Check sheet for the modelled part. Datum: model origin and axes. Units: mm. A direction names the side the tool comes from. Round coordinates to 2 decimals unless told otherwise and drop trailing zeros. Loops run counter-clockwise (first coordinate to the right, second up) from the corner with the lowest first, then second, coordinate; pieces in that order, holes last. Notation, with made-up numbers: (16, 31.5) -> (64, 31.5) arc R21 ccw to (64, 50.5) -> close; hole circle Ø7 at (24, -31). An arc over 180 degrees is marked (long way). Use one line per item in the form item = value. Start each with the question number.
(1) Go/stop test with flat-tipped pins: pin 1 (5 mm diameter, centred on y = -17.5, z = 2, fed in from +X); pin 2 (10 mm diameter, centred on x = 4, y = 0, fed in from -Z); pin 3 (4.5 mm diameter, centred on x = 78, y = 8.94, fed in from -Z). Record where each tip stops, or that it passes through.
(2) Draft check along Y on faces 1 (the flat face through (23, -18, 0)), 2 (the flat face through (77, -27.6, 4)), 3 (the cylindrical face through (80.747, -19.279, 8.433)). Enter one of: released by +Y, released by -Y, zero draft, split by the parting line, or undercut.
(3) Material ranges on probe 1 along Y at (x, z) = (4, 10.15); probe 2 along X at (y, z) = (-8.5, 3); probe 3 along Y at (x, z) = (4, 8.2), recorded low to high. Write a range as [from, to].
(4) Sectioned sample at D-D (x = 37.5). Record the cut outline in (y, z), and give its area (3 significant figures).
(5) Set-up check for faces 4 (the flat face through (52.85, -31, 2)), 5 (the cylindrical face through (58.969, 2.047, 0.805)), 6 (the flat face through (24.25, -10, 2)), 7 (the flat face through (6, -8, 7.25)), 8 (the flat face through (66.25, -10, 2)): record each of +Z, -Z, +X, -X, +Y, -Y from which the full face is reachable in a straight line by a thin tool's end or side.
(6) Sectioned sample at A-A (y = -14.5). Record the cut outline in (x, z) (3 decimals), and give its area (3 significant figures).
(7) Sectioned sample at B-B (x = 20). Record the cut outline in (y, z), and give its area (3 significant figures).
(8) Sectioned sample at C-C (z = 8.5). Record the cut outline in (x, y), and give its area (3 significant figures).
from build123d import *

# Parameters (mm, degrees)
SKETCH1_R                = 1.6
BOSS_EXTRUDE1_DEPTH      = 11.15
SKETCH2_W                = 82
SKETCH2_H                = 0.6
CUT_EXTRUDE1_DEPTH       = 8
CUT_EXTRUDE2_DEPTH       = 46.2
CUT_EXTRUDE3_DEPTH       = 40.2
CUT_EXTRUDE5_DEPTH       = 39.2
BOSS_EXTRUDE2_DEPTH      = 32.2
CHAMFER3_SIZE            = 1.1
CHAMFER4_SIZE            = 1.1
CUT_EXTRUDE12_DEPTH      = 1
CUT_EXTRUDE12_DEPTH_BACK = 83
FILLET3_R                = 15
SKETCH14_R               = 1.6
CUT_EXTRUDE14_DEPTH      = 12.1500001
BOSS_EXTRUDE3_DEPTH      = 3.5
SKETCH8_W                = 82
SKETCH8_H                = 0.6
CUT_EXTRUDE16_DEPTH      = 4.15
SKETCH20_R               = 2.75
CUT_EXTRUDE17_DEPTH      = 2.4
CHAMFER5_SIZE            = 0.5


with BuildPart() as part:
    # Sketch1 → Boss-Extrude1 (new body)
    with BuildSketch(Plane.XY):
        with BuildLine():
            Line((0, -35.2), (82, -35.2))
            Line((82, -35.2), (82, 8.75))
            ThreePointArc((82, 8.75), (81.165254326, 10.765254326), (79.15, 11.6))
            Line((79.15, 11.6), (2.85, 11.6))
            ThreePointArc((2.85, 11.6), (0.834745674, 10.765254326), (0, 8.75))
            Line((0, 8.75), (0, -35.2))
        make_face()
        with Locations((4, 8.939640599)):
            Circle(SKETCH1_R, mode=Mode.SUBTRACT)
        with Locations((78, 8.939640599)):
            Circle(SKETCH1_R, mode=Mode.SUBTRACT)
    extrude(amount=BOSS_EXTRUDE1_DEPTH)

    # Sketch2 → Cut-Extrude1 (cut)
    with BuildSketch(Plane(origin=(0, 0, 0), x_dir=(-1, 0, 0), z_dir=(0, 0, -1))):
        with Locations((-41, -34.9)):
            Rectangle(SKETCH2_W, SKETCH2_H)
    cut_extrude1 = extrude(amount=-CUT_EXTRUDE1_DEPTH, mode=Mode.SUBTRACT)

    # Sketch3 → Cut-Extrude2 (cut)
    with BuildSketch(Plane.XZ.offset(34.6)):
        with BuildLine():
            Line((25.85, 4), (25.85, 0))
            Line((25.85, 0), (29.15, 0))
            Line((29.15, 0), (29.15, 4))
            ThreePointArc((29.15, 4), (27.5, 5.65), (25.85, 4))
        make_face()
        with BuildLine():
            ThreePointArc((14.15, 4), (12.5, 5.65), (10.85, 4))
            Line((10.85, 4), (10.85, 0))
            Line((10.85, 0), (14.15, 0))
            Line((14.15, 0), (14.15, 4))
        make_face()
        with BuildLine():
            ThreePointArc((23.25, 4), (20, 7.25), (16.75, 4))
            Line((16.75, 4), (16.75, 0))
            Line((16.75, 0), (23.25, 0))
            Line((23.25, 0), (23.25, 4))
        make_face()
    cut_extrude2 = extrude(amount=-CUT_EXTRUDE2_DEPTH, mode=Mode.SUBTRACT)

    # Sketch4 → Cut-Extrude3 (cut)
    with BuildSketch(Plane(origin=(0, 11.6, 0), x_dir=(1, 0, 0), z_dir=(0, 1, 0))):
        with BuildLine():
            Line((9.25, -4), (9.25, 0))
            Line((9.25, 0), (15.75, 0))
            Line((15.75, 0), (15.75, -4))
            ThreePointArc((15.75, -4), (12.5, -7.25), (9.25, -4))
        make_face()
        with BuildLine():
            Line((24.25, -4), (24.25, 0))
            Line((24.25, 0), (30.75, 0))
            Line((30.75, 0), (30.75, -4))
            ThreePointArc((30.75, -4), (27.5, -7.25), (24.25, -4))
        make_face()
    cut_extrude3 = extrude(amount=-CUT_EXTRUDE3_DEPTH, mode=Mode.SUBTRACT)

    # Sketch6 → Cut-Extrude5 (cut)
    with BuildSketch(Plane(origin=(0, 11.6, 0), x_dir=(1, 0, 0), z_dir=(0, 1, 0))):
        with BuildLine():
            Line((15.75, -4), (15.75, 0))
            Line((15.75, 0), (15.75, 1.061213364))
            Line((15.75, 1.061213364), (0, 1.061213364))
            Line((0, 1.061213364), (0, -7.25))
            Line((0, -7.25), (12.5, -7.25))
            ThreePointArc((12.5, -7.25), (14.798097039, -6.298097039), (15.75, -4))
        make_face()
        with BuildLine():
            Line((24.25, 0), (24.25, -4))
            ThreePointArc((24.25, -4), (25.201902961, -6.298097039), (27.5, -7.25))
            Line((27.5, -7.25), (41, -7.25))
            Line((41, -7.25), (41, 0))
            Line((41, 0), (24.25, 0))
        make_face()
    cut_extrude5 = extrude(amount=-CUT_EXTRUDE5_DEPTH, mode=Mode.SUBTRACT)

    # Mirror1: Cut-Extrude1, Cut-Extrude2, Cut-Extrude3, Cut-Extrude5 across plane
    add(cut_extrude1.mirror(Plane.ZY.offset(-41)), mode=Mode.SUBTRACT)
    add(cut_extrude2.mirror(Plane.ZY.offset(-41)), mode=Mode.SUBTRACT)
    add(cut_extrude3.mirror(Plane.ZY.offset(-41)), mode=Mode.SUBTRACT)
    add(cut_extrude5.mirror(Plane.ZY.offset(-41)), mode=Mode.SUBTRACT)

    # Sketch12 → Boss-Extrude2 (add)
    with BuildSketch(Plane(origin=(0, 11.6, 0), x_dir=(1, 0, 0), z_dir=(0, 1, 0))):
        with BuildLine():
            Line((16.75, -4), (16.75, 0))
            Line((16.75, 0), (18, 0))
            Line((18, 0), (18.11, -3.084631222))
            ThreePointArc((18.11, -3.084631222), (20, -6.1), (21.89, -3.084631222))
            Line((21.89, -3.084631222), (22, 0))
            Line((22, 0), (23.25, 0))
            Line((23.25, 0), (23.25, -4))
            ThreePointArc((23.25, -4), (20, -7.25), (16.75, -4))
        make_face()
        with BuildLine():
            Line((58.75, -4), (58.75, 0))
            Line((58.75, 0), (60.05, 0))
            Line((60.05, 0), (60.155, -3.106425717))
            ThreePointArc((60.155, -3.106425717), (62, -6.05), (63.845, -3.106425717))
            Line((63.845, -3.106425717), (63.95, 0))
            Line((63.95, 0), (65.25, 0))
            Line((65.25, 0), (65.25, -4))
            ThreePointArc((65.25, -4), (62, -7.25), (58.75, -4))
        make_face()
    extrude(amount=-BOSS_EXTRUDE2_DEPTH)

    # Chamfer3
    chamfer3_edges = [part.edges().sort_by_distance(p)[0] for p in [
        (65.25, -20.6, 2),
        (58.75, -20.6, 2),
        (62, -20.6, 7.25),
    ]]
    chamfer(chamfer3_edges, length=CHAMFER3_SIZE)

    # Chamfer4
    chamfer4_edges = [part.edges().sort_by_distance(p)[0] for p in [
        (23.25, -20.6, 2),
        (16.75, -20.6, 2),
        (20, -20.6, 7.25),
    ]]
    chamfer(chamfer4_edges, length=CHAMFER4_SIZE)

    # Sketch9 → Cut-Extrude12 (cut, two sides)
    with BuildSketch(Plane.ZY) as cut_extrude12_sk:
        Polygon((-106.219800457, 11.6), (0, 11.6), (7.25, 11.6), (0, 2.4), (-65.744961499, -81.028089075), (-260.411588221, -166.089763625), (-300.886427179, -73.46167455), align=None)
    extrude(amount=CUT_EXTRUDE12_DEPTH, mode=Mode.SUBTRACT)
    extrude(cut_extrude12_sk.sketch, amount=-CUT_EXTRUDE12_DEPTH_BACK, mode=Mode.SUBTRACT)

    # Fillet3
    fillet3_edges = [part.edges().sort_by_distance(p)[0] for p in [
        (16.875, 2.4, 0),
        (23.125, 2.4, 0),
        (58.9, 2.4, 0),
        (65.1, 2.4, 0),
    ]]
    fillet(fillet3_edges, radius=FILLET3_R)

    # Sketch14 → Cut-Extrude14 (cut, through all)
    with BuildSketch(Plane.XY.offset(11.15)):
        with Locations((4, -19.400359401)):
            Circle(SKETCH14_R)
    cut_extrude14 = extrude(amount=-CUT_EXTRUDE14_DEPTH, mode=Mode.SUBTRACT)

    # Mirror3: Cut-Extrude14 across plane
    add(cut_extrude14.mirror(Plane.ZY.offset(-41)), mode=Mode.SUBTRACT)

    # Sketch18 → Boss-Extrude3 (add)
    with BuildSketch(Plane(origin=(0, -27.6, 0), x_dir=(1, 0, 0), z_dir=(0, 1, 0))):
        with BuildLine():
            Line((14.15, 0), (14.15, -1.2))
            ThreePointArc((14.15, -1.2), (15.321790212, -2.38754845), (15.75, -4))
            Line((15.75, -4), (15.75, 0))
            Line((15.75, 0), (14.15, 0))
        make_face()
        with BuildLine():
            Line((10.85, -1.2), (10.85, 0))
            Line((10.85, 0), (9.25, 0))
            Line((9.25, 0), (9.25, -4))
            ThreePointArc((9.25, -4), (9.678209788, -2.38754845), (10.85, -1.2))
        make_face()
        with BuildLine():
            Line((29.15, 0), (29.15, -1.2))
            ThreePointArc((29.15, -1.2), (30.321790212, -2.38754845), (30.75, -4))
            Line((30.75, -4), (30.75, 0))
            Line((30.75, 0), (29.15, 0))
        make_face()
        with BuildLine():
            Line((25.85, -1.2), (25.85, 0))
            Line((25.85, 0), (24.25, 0))
            Line((24.25, 0), (24.25, -4))
            ThreePointArc((24.25, -4), (24.678209788, -2.38754845), (25.85, -1.2))
        make_face()
    boss_extrude3 = extrude(amount=-BOSS_EXTRUDE3_DEPTH)

    # Mirror5: Boss-Extrude3 across plane
    add(boss_extrude3.mirror(Plane.ZY.offset(-41)))

    # Sketch8 → Cut-Extrude16 (cut, through all)
    with BuildSketch(Plane(origin=(0, 0, 8), x_dir=(-1, 0, 0), z_dir=(0, 0, -1))):
        with Locations((-41, -34.9)):
            Rectangle(SKETCH8_W, SKETCH8_H)
    extrude(amount=-CUT_EXTRUDE16_DEPTH, mode=Mode.SUBTRACT)

    # Sketch20 → Cut-Extrude17 (cut)
    with BuildSketch(Plane(origin=(0, 0, 7.25), x_dir=(-1, 0, 0), z_dir=(0, 0, -1))):
        with Locations((-78, 8.939640599)):
            Circle(SKETCH20_R)
        with Locations((-78, -19.400359401)):
            Circle(SKETCH20_R)
    cut_extrude17 = extrude(amount=-CUT_EXTRUDE17_DEPTH, mode=Mode.SUBTRACT)

    # Mirror7: Cut-Extrude17 across plane
    add(cut_extrude17.mirror(Plane.ZY.offset(-41)), mode=Mode.SUBTRACT)

    # Chamfer5
    chamfer5_edges = [part.edges().sort_by_distance(p)[0] for p in [
        (2.4, 8.939640599, 11.15),
        (76.4, 8.939640599, 11.15),
        (2.4, -19.400359401, 11.15),
        (79.6, -19.400359401, 11.15),
    ]]
    chamfer(chamfer5_edges, length=CHAMFER5_SIZE)


solid = part.part
Checks:
q1.pin_1 = 66.29
q1.pin_2 = 7.25
q1.pin_3 = 9.65
q2.face_1 = zero draft
q2.face_2 = released by +Y
q2.face_3 = undercut
q3.probe_1 = [-34.6, -21], [-17.8, 7.34], [10.54, 11.6]
q3.probe_2 = [15.75, 18.11], [21.89, 24.25], [57.75, 60.15], [63.85, 66.25]
q3.probe_3 = [-34.6, -22.15], [-16.65, 6.19]
q4.outline = (-34.6, 0) -> (-27.6, 0) -> (-27.6, 7.25) -> (11.6, 7.25) -> (11.6, 11.15) -> (-34.6, 11.15) -> close
q4.area = 231 mm2
q5.face_4 = -Z, +Y, -Y
q5.face_5 = -Z, +X, -X, +Y
q5.face_6 = -Z, +Y
q5.face_7 = -Z, -X, +Y
q5.face_8 = -Z, +X, +Y
q6.outline = (0, 7.25) -> (12.5, 7.25) arc R3.25 cw to (15.75, 4) -> (15.75, 0) -> (18, 0) -> (18.11, 3.085) arc R2.1 cw (long way) to (21.89, 3.085) -> (22, 0) -> (24.25, 0) -> (24.25, 4) arc R3.25 cw to (27.5, 7.25) -> (54.5, 7.25) arc R3.25 cw to (57.75, 4) -> (57.75, 0) -> (60.05, 0) -> (60.155, 3.106) arc R2.05 cw (long way) to (63.845, 3.106) -> (63.95, 0) -> (66.25, 0) -> (66.25, 4) arc R3.25 cw to (69.5, 7.25) -> (82, 7.25) -> (82, 11.15) -> (0, 11.15) -> close
q6.area = 408 mm2
q7.outline = (-34.6, 7.25) -> (-21.7, 7.25) -> (-20.6, 6.15) -> (-20.6, 6.1) -> (10.14, 6.1) -> (11.6, 7.25) -> (11.6, 11.15) -> (-34.6, 11.15) -> close
q7.area = 217 mm2
q8.outline = (0, -34.6) -> (82, -34.6) -> (82, 8.75) arc R2.85 ccw to (79.15, 11.6) -> (78.7, 11.6) arc R2.75 cw (long way) to (77.3, 11.6) -> (4.7, 11.6) arc R2.75 cw (long way) to (3.3, 11.6) -> (2.85, 11.6) arc R2.85 ccw to (0, 8.75) -> close; hole circle Ø5.5 at (4, -19.4); hole circle Ø5.5 at (78, -19.4)
q8.area = 3,690 mm2
